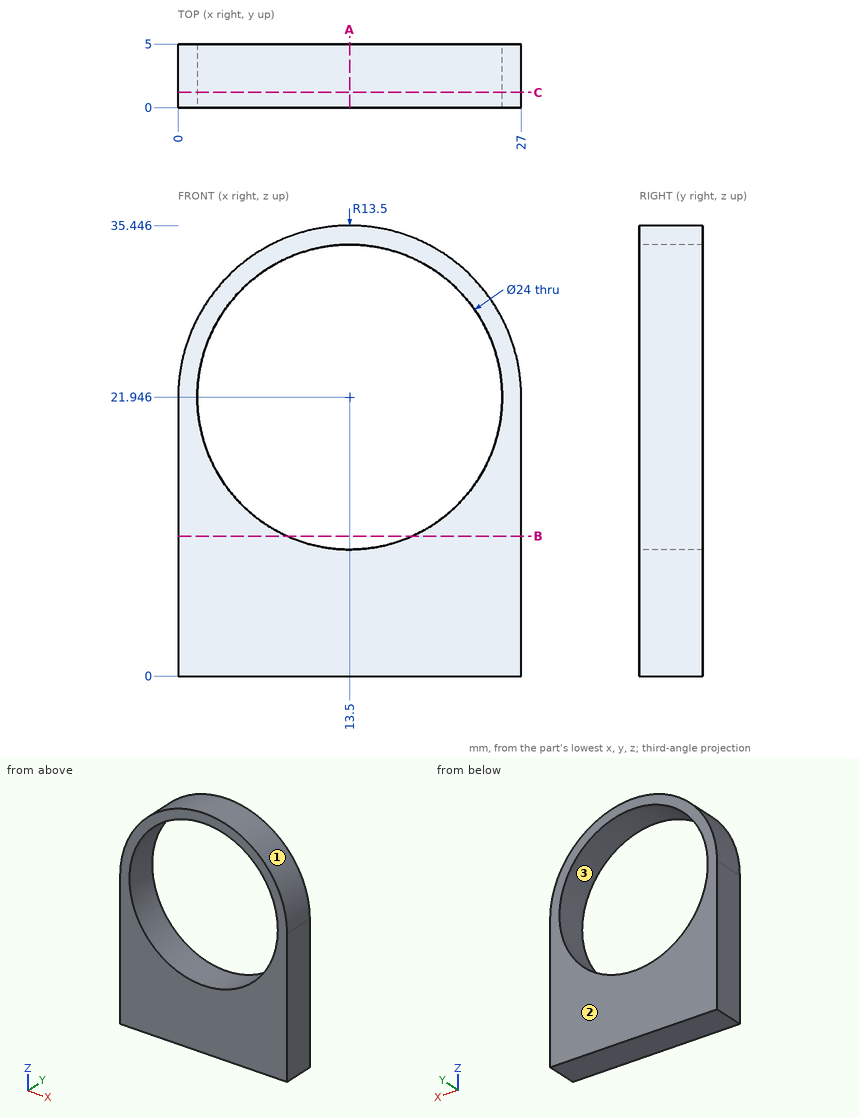
Study the drawing (mm; zero at the part's minimum x, y, z) and answer. Give positions to 0.01 mm unless a question says otherwise; leave off trailing zeros. Write each loop counter-clockwise with the first axis right and the second up, starting at its lowest first coordinate (ties: lowest second). Pieces come first, ordered by that corner, then holes. Notation, with made-up numbers: (75.5, 25) -> (127.5, 25) arc R25 cw to (127.5, 42) -> close; hole circle Ø5 at (12, 56.25). An arc over 180 degrees is marked (long way). Write item = value, one per line. Start each with the question number.
1) Straight lines are drawn through the part: line 1 along X through (y, z) = (3.5, 21.5); line 2 along Z through (x, y) = (13.75, 4.4); line 3 along Z through (x, y) = (21, 1.25). For each, find the intervals that lie inside material, in ascending order.
2) The part is cut by section C-C, the plane y = 1.2. Determine the outline of the cut face in (x, z), and give its area (3 significant figures).
3) Each of these flat-tipped pins is pushed along its axis until it touches: pin 1 (1.5 mm diameter, centred on x = 4.5, y = 1, fed in from +Z); pin 2 (1 mm diameter, centred on y = 4.5, z = 27.5, fed in from -X); pin 3 (2 mm diameter, centred on y = 2.5, z = 23.5, fed in from +X). Where does it stop, or does it pass through?
4) Determine the mould class of the marked faces 1, 2 and 3 for opening direction Z: +Z half, -Z half, draft (parallel to the pull), parting line (faces both ways), or undercut.
5) The part is cut by section B-B, the plane z = 11. Determine the outline of the cut face in (x, y), and give its area (3 significant figures).
6) The part is cut by section A-A, the plane x = 13.5. Determine the outline of the cut face in (y, z).
Solutions:
q1.line_1 = 0 to 1.51, 25.49 to 27
q1.line_2 = 0 to 9.95, 33.94 to 35.44
q1.line_3 = 0 to 12.58, 31.31 to 33.17
q2.outline = (0, 0) -> (27, 0) -> (27, 21.95) arc R13.5 ccw to (0, 21.95) -> close; hole circle Ø24 at (13.5, 21.95)
q2.area = 426 mm²
q3.pin_1 = 32.63
q3.pin_2 = 0.98
q3.pin_3 = 26.99
q4.face_1 = +Z half
q4.face_2 = draft
q4.face_3 = undercut
q5.outline = (0, 0) -> (8.58, 0) -> (8.58, 5) -> (0, 5) -> close; (18.42, 0) -> (27, 0) -> (27, 5) -> (18.42, 5) -> close
q5.area = 85.8 mm²
q6.outline = (0, 0) -> (5, 0) -> (5, 9.95) -> (0, 9.95) -> close; (0, 33.95) -> (5, 33.95) -> (5, 35.45) -> (0, 35.45) -> close
